CAD build for the part. Positions are in the model's coordinates, mm. Coordinates: 2 decimals unless noted, no trailing zeros. Write each loop counter-clockwise with the first axis right and the second up, starting at its lowest first coordinate (ties: lowest second). Pieces come first, ordered by that corner, then holes. Notation, with made-up numbers: (39.25, 87) - (79.25, 87) arc R26 ccw to (79.25, 114) - close; hole circle Ø4 at (6.25, 46.25). An arc over 180 degrees is marked (long way). One line per question, with ' | ' between items. Start each with the question number.
1. Flat gauge pin, fed straight in: P1, Ø1.5, axis at y = 1.5, z = 1, coming from the +X side. Where does the tip first touch, or does it go through?
2. Probe line 1 (Z direction, x = 0, y = 2.3) (3 decimals); line 2 (Z direction, x = 13, y = 4); line 3 (X direction, y = 0.7, z = -5.5). List the from-to ranges inside material, lowest first.
3. Band-saw the part on D-D, the plane z = 6. Write the cut outline in (x, y), then the cut area to 3 significant figures.
4. Band-saw the part on B-B, the plane z = 0. Write the cut outline in (x, y).
5. Band-saw the part on A-A, the plane y = 3. Write the cut outline in (x, z) (3 decimals), then the cut area to 3 significant figures.
6. Two-plate mould, pull along Z, no slides. Class faces 1 (the cylindrical face through (-13.887, 2.218, -10.648)), 2 (the cylindrical face through (-2.17, 2.22, -9.76)), 3 (the flat face through (8, 4.5, 8)): +Z half, -Z half, draft (parallel to the pull), parting line (faces both ways), or undercut.
7. Band-saw the part on C-C, the plane x = 0. Write the cut outline in (y, z) (3 decimals).
from build123d import *

# Parameters (mm, degrees)
SKETCH_1_R               = 31.5
SKETCH_1_R_2             = 22.5
EXTRUDE_1_DEPTH          = 4.5
SKETCH_2_R               = 2.025
CUT_EXTRUDE_1_DEPTH      = 1
CUT_EXTRUDE_1_DEPTH_BACK = 5.5
SKETCH_3_R               = 22.5
EXTRUDE_2_DEPTH          = 4.5
SKETCH_4_R               = 1.525
CUT_EXTRUDE_2_DEPTH      = 4.5
SKETCH_5_R               = 10
CUT_EXTRUDE_3_DEPTH      = 4.5
SKETCH_6_R               = 31.5
SKETCH_6_R_2             = 17.5
CUT_EXTRUDE_4_DEPTH      = 5.5


with BuildPart() as part:
    # 草图1 → 凸台-拉伸1 (new body)
    with BuildSketch(Plane(origin=(0, 0, 0), x_dir=(1, 0, 0), z_dir=(0, 1, 0))):
        Circle(SKETCH_1_R)
        Circle(SKETCH_1_R_2, mode=Mode.SUBTRACT)
    extrude(amount=EXTRUDE_1_DEPTH)

    # 草图2 → 切除-拉伸1 (cut, two sides)
    with BuildSketch(Plane(origin=(0, 4.5, 0), x_dir=(1, 0, 0), z_dir=(0, 1, 0))) as cut_extrude_1_sk:
        with Locations((0, 26.25)):
            Circle(SKETCH_2_R)
        with Locations((18.561553006, 18.561553006)):
            Circle(SKETCH_2_R)
        with Locations((26.25, 0)):
            Circle(SKETCH_2_R)
        with Locations((18.561553006, -18.561553006)):
            Circle(SKETCH_2_R)
        with Locations((0, -26.25)):
            Circle(SKETCH_2_R)
        with Locations((-18.561553006, -18.561553006)):
            Circle(SKETCH_2_R)
        with Locations((-26.25, 0)):
            Circle(SKETCH_2_R)
        with Locations((-18.561553006, 18.561553006)):
            Circle(SKETCH_2_R)
    extrude(amount=CUT_EXTRUDE_1_DEPTH, mode=Mode.SUBTRACT)
    extrude(cut_extrude_1_sk.sketch, amount=-CUT_EXTRUDE_1_DEPTH_BACK, mode=Mode.SUBTRACT)

    # 草图3 → 凸台-拉伸2 (add)
    with BuildSketch(Plane(origin=(0, 4.5, 0), x_dir=(1, 0, 0), z_dir=(0, 1, 0))):
        Circle(SKETCH_3_R)
    extrude(amount=-EXTRUDE_2_DEPTH)

    # 草图4 → 切除-拉伸2 (cut)
    with BuildSketch(Plane.XZ):
        with Locations((0, 13.5)):
            Circle(SKETCH_4_R)
        with Locations((11.691342951, 6.75)):
            Circle(SKETCH_4_R)
        with Locations((11.691342951, -6.75)):
            Circle(SKETCH_4_R)
        with Locations((0, -13.5)):
            Circle(SKETCH_4_R)
        with Locations((-11.691342951, -6.75)):
            Circle(SKETCH_4_R)
        with Locations((-11.691342951, 6.75)):
            Circle(SKETCH_4_R)
    extrude(amount=-CUT_EXTRUDE_2_DEPTH, mode=Mode.SUBTRACT)

    # 草图5 → 切除-拉伸3 (cut)
    with BuildSketch(Plane.XZ):
        Circle(SKETCH_5_R)
    extrude(amount=-CUT_EXTRUDE_3_DEPTH, mode=Mode.SUBTRACT)

    # 草图6 → 切除-拉伸4 (cut, through all)
    with BuildSketch(Plane.XZ):
        Circle(SKETCH_6_R)
        Circle(SKETCH_6_R_2, mode=Mode.SUBTRACT)
    extrude(amount=-CUT_EXTRUDE_4_DEPTH, mode=Mode.SUBTRACT)


solid = part.part
Filled in:
1) P1: stops at x = 17.5
2) line 1: z = -17.5 to -15.025, -11.975 to -10, 10 to 11.975, 15.025 to 17.5 | line 2: z = -11.72 to -7.53, -5.97 to 5.97, 7.53 to 11.72 | line 3: x = -16.61 to -12.56, -10.82 to -8.35, 8.35 to 10.82, 12.56 to 16.61
3) outline: (-16.44, 0) - (-13.02, 0) - (-13.02, 4.5) - (-16.44, 4.5) - close; (-10.36, 0) - (-8, 0) - (-8, 4.5) - (-10.36, 4.5) - close; (8, 0) - (10.36, 0) - (10.36, 4.5) - (8, 4.5) - close; (13.02, 0) - (16.44, 0) - (16.44, 4.5) - (13.02, 4.5) - close | area: 52.1 mm²
4) outline: (-17.5, 0) - (-10, 0) - (-10, 4.5) - (-17.5, 4.5) - close; (10, 0) - (17.5, 0) - (17.5, 4.5) - (10, 4.5) - close
5) outline: circle Ø35 at (0, 0); hole circle Ø3.05 at (-11.691, -6.75); hole circle Ø3.05 at (-11.691, 6.75); hole circle Ø20 at (0, 0); hole circle Ø3.05 at (0, -13.5); hole circle Ø3.05 at (0, 13.5); hole circle Ø3.05 at (11.691, -6.75); hole circle Ø3.05 at (11.691, 6.75) | area: 604 mm²
6) face 1: parting line | face 2: undercut | face 3: draft
7) outline: (0, -17.5) - (4.5, -17.5) - (4.5, -15.025) - (0, -15.025) - close; (0, -11.975) - (4.5, -11.975) - (4.5, -10) - (0, -10) - close; (0, 10) - (4.5, 10) - (4.5, 11.975) - (0, 11.975) - close; (0, 15.025) - (4.5, 15.025) - (4.5, 17.5) - (0, 17.5) - close
